Geometry check sheet. Reference: the model listing, model coordinates, mm. A direction names the side the tool comes from. Give positions to 0.01 mm unless a question says otherwise; leave off trailing zeros. Write each loop counter-clockwise with the first axis right and the second up, starting at its lowest first coordinate (ties: lowest second). Pieces come first, ordered by that corner, then holes.
(1) Thickness scan on line 1 along X through (y, z) = (1.55, 10); line 2 along Z through (x, y) = (5, 2.8); line 3 along Y through (x, z) = (7.25, 7.25). Record the ranges inside material, lowest first.
(2) Mould release check, pull along X, two halves, no side actions. Record for faces 3 (the flat face through (10, 6, 4)), 4 (the cylindrical face through (5.07, 5.57, 5.6)), 5 (the cylindrical face through (6.386, 9.425, 2.535)): +X half, -X half, draft (parallel to the pull), parting line (faces both ways), or undercut.
(3) Cross-section at A-A (y = 10). Record the boundary of the cut face in (x, z).
(4) Tool access check on faces 1 (the flat face through (3.8, 5, 11.3)), 2 (the flat face through (4.9, 2.5, 15)). Record the directions out of +Z, -Z, +X, -X, +Y, -Y that give a thin tool (end or side, any length) a straight path to the whole face; none if there is none.
(5) Depth check by flat-ended pin: P1, Ø4, axis at x = 5, z = 10, coming from the +Y side; P2, Ø4, axis at x = 5, y = 10, coming from the +Z side; P3, Ø1.5, axis at y = 6.5, z = 10.5, coming from the -X side. Enter the tip coordinate at first touch or a pass-through.
(6) Cross-section at D-D (x = 7.5). Record the boundary of the cut face in (y, z), and give its area (3 significant figures).
(7) Cross-section at C-C (x = 5). Record the boundary of the cut face in (y, z).
Autodesk Inventor part; units mm, degrees
ref_plane "YZ Plane" through (0, 0, 0) normal (1, 0, 0) x (0, 1, 0)
ref_plane "XZ Plane" through (0, 0, 0) normal (0, 1, 0) x (-1, 0, 0)
ref_plane "XY Plane" through (0, 0, 0) normal (0, 0, 1) x (1, 0, 0)
sketch "Sketch1" plane through (0, 0, 0) normal (1, 0, 0) x (0, 1, 0)
  line L0 (0, 0) -> (5, 0)
  line L1 (5, 5) -> (5, 15)
  line L2 (5, 15) -> (0, 15)
  line L3 (0, 15) -> (0, 0)
  line L4 (0, 0) -> (15, 0)
  line L5 (15, 0) -> (15, 5)
  line L6 (15, 5) -> (5, 5)
  line L7 (0, 15) -> (0, 0)
  point P0 (2.5, 15)
  point P1 (2.5, 0)
  point P2 (0, 7.5)
  point P3 (15, 2.5)
  dimension "d0" = 15
  dimension "d2" = 10
  dimension "d3" = 10
  dimension "d4" = 15
  dimension "d5" = 5
  dimension "d6" = 10
extrude "Extrusion1" add sketch "Sketch1" along normal blind 10
fillet "Fillet1" radius 2 6 edges at (5, 5, 5) (5, 0, 0) (5, 5, 15) (5, 0, 15) (5, 15, 5) (5, 15, 0)
sketch "Sketch2" plane through (0, 5, 13) normal (0, 1, 0) x (1, 0, 0)
  circle A0 centre (5, 3) radius 1.5
  line L0 (0, 6) -> (0, 0)
  line L1 (0, -2) -> (10, -2)
  point P0 (0, 13)
  point P1 (5, -2)
  dimension "d10" = 5
  dimension "d11" = 5
  dimension "d12" = 3
sketch "Sketch3" plane through (0, 7, 5) normal (0, 0, 1) x (1, 0, 0)
  circle A0 centre (5, 3) radius 1.5
  line L0 (10, 8) -> (0, 8)
  line L1 (0, 6) -> (0, 0)
  point P0 (0, -7)
  point P1 (5, 8)
  point P2 (0, 3)
  dimension "d13" = 3
  dimension "d14" = 5
  dimension "d15" = 5
extrude "Extrusion2" cut sketch "Sketch2" against normal through all
extrude "Extrusion3" cut sketch "Sketch3" against normal through all
properties part number "L joint"
Reply:
1. line 1: x = 0 to 3.5, 6.5 to 10
1. line 2: z = 0 to 8.5, 11.5 to 15
1. line 3: y = 0 to 5
2. face 3: +X half
2. face 4: draft
2. face 5: undercut
3. outline: (0, 0) - (3.5, 0) - (3.5, 5) - (0, 5) - close; (6.5, 0) - (10, 0) - (10, 5) - (6.5, 5) - close
4. face 1: +Z, +X, -X, +Y
4. face 2: +Z, +X, -X, +Y, -Y
5. P1: stops at y = 5
5. P2: stops at z = 5
5. P3: passes through
6. outline: (0, 2) arc R2 ccw to (2, 0) - (13, 0) arc R2 ccw to (15, 2) - (15, 3) arc R2 ccw to (13, 5) - (7, 5) arc R2 cw to (5, 7) - (5, 13) arc R2 ccw to (3, 15) - (2, 15) arc R2 ccw to (0, 13) - close
6. area: 122 mm2
7. outline: (0, 2) arc R2 ccw to (2, 0) - (8.5, 0) - (8.5, 5) - (7, 5) arc R2 cw to (5, 7) - (5, 8.5) - (0, 8.5) - close; (0, 11.5) - (5, 11.5) - (5, 13) arc R2 ccw to (3, 15) - (2, 15) arc R2 ccw to (0, 13) - close; (11.5, 0) - (13, 0) arc R2 ccw to (15, 2) - (15, 3) arc R2 ccw to (13, 5) - (11.5, 5) - close
